Build history of the part. All positions in model axes, mm. Face numbers are marked on the shaded views. A direction names the side the tool comes from. Round coordinates to 2 decimals unless told otherwise and drop trailing zeros. Order: outer loops, then holes, each group sorted by start corner. A loop starts at its lowest first (then second) coordinate and runs counter-clockwise, first axis right, second up. Notation, with made-up numbers: (53, 41) -> (66, 41) arc R17 cw to (66, 51) -> close; hole circle Ø11 at (72, 21). An arc over 180 degrees is marked (long way). Write item = value, one per line.
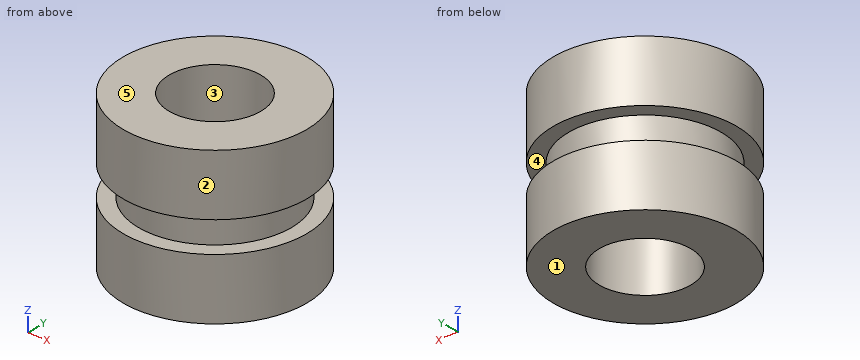
from build123d import *

# Parameters (mm, degrees)
F0_R     = 2.5
F0_R_2   = 1.5
F1_DEPTH = 5
F0_R_3   = 3
F2_DEPTH = 2
F3_R     = 3
F3_R_2   = 2.5
F4_DEPTH = 2


with BuildPart() as f1:
    # F0 (on Top) → F1 (new body)
    with BuildSketch(Plane.XY):
        Circle(F0_R)
        Circle(F0_R_2, mode=Mode.SUBTRACT)
    extrude(amount=F1_DEPTH)

    # F0 (on Top) → F2 (join)
    with BuildSketch(Plane.XY):
        Circle(F0_R_3)
        Circle(F0_R, mode=Mode.SUBTRACT)
    extrude(amount=F2_DEPTH)

    # F3 (on face) → F4 (join)
    with BuildSketch(Plane.XY.offset(5)):
        Circle(F3_R)
        Circle(F3_R_2, mode=Mode.SUBTRACT)
    extrude(amount=-F4_DEPTH)


solid = f1.part
Q1. Mould opens along X. For the marked faces 1, 2 and 3 say: released by +X, released by -X, zero draft, split by the parting line, or undercut.
Check values:
face_1 = zero draft
face_2 = split by the parting line
face_3 = undercut
Q2. Flat gauge pins, fed straight in: pin 1 (2 mm diameter, centred on y = -1.5, z = 0.5, fed in from -X); pin 2 (1.8 mm diameter, centred on x = 0, y = 0, fed in from -Z). Where does each tip first touch, or does it go through?
Check values:
pin_1 = -2.96
pin_2 = through
Q3. Which spindle directions (+Z, -Z, +X, -X, +Y, -Y) get a long thin tool onto all of the face, cutting with end or side? Do the marked faces 4 and 5. Say none if no direction does.
Check values:
face_4 = none
face_5 = +Z, +X, -X, +Y, -Y
Q4. Cut at A-A, the plane y = 0. List the corners of the cut face in (x, z).
Check values:
outline = (-3, 0) -> (-1.5, 0) -> (-1.5, 5) -> (-3, 5) -> (-3, 3) -> (-2.5, 3) -> (-2.5, 2) -> (-3, 2) -> close; (1.5, 0) -> (3, 0) -> (3, 2) -> (2.5, 2) -> (2.5, 3) -> (3, 3) -> (3, 5) -> (1.5, 5) -> close
Q5. Probe probe 1 along Z at (x, y) = (-1.2, 2.3); probe 2 along Y at (x, z) = (0, 3.85); probe 3 along Y at (x, z) = (0.15, 2.4). List the from-to ranges inside material, lowest first.
Check values:
probe_1 = 0 to 2, 3 to 5
probe_2 = -3 to -1.5, 1.5 to 3
probe_3 = -2.5 to -1.49, 1.49 to 2.5
Q6. Cut at C-C, the plane z = 0.55. List the corners of the cut face in (x, y).
Check values:
outline = circle Ø6 at (0, 0); hole circle Ø3 at (0, 0)
